Input: part model. Units: mm. Frame: model coordinates. Round coordinates to 2 decimals unless told otherwise and drop trailing zeros. Loops run counter-clockwise (first coordinate to the right, second up) from the corner with the lowest first, then second, coordinate; pieces in that order, holes last.
(1) Line query: line 1 (Y direction, x = -32, z = 10.75) (3 decimals); line 2 (Z direction, x = -163, y = -204); line 3 (Y direction, x = -152.5, z = 1) (3 decimals). Output: solid intervals per line, ascending.
(2) First-contact query: pin 1 Ø16 at (x, y) = (-15.92, -195.49) entering from -Z; pin 2 Ø3 at (x, y) = (-34, -167.5) entering from +Z; pin 3 Ø6.5 at (x, y) = (-86.2, -169.85) entering from +Z. Flat tips, straight axial feed; report the tip coordinate or a pass-through.
(3) Cut plane A-A, the plane x = -124.32. Output: boundary loops of the cut face in (y, z) (3 decimals), and give its area (3 significant figures).
from build123d import *

# Parameters (mm, degrees)
SKETCH1_W                                      = 184.15
SKETCH1_H                                      = 146.05
BOSS_EXTRUDE1_DEPTH                            = 12.7
SKETCH5_W                                      = 184.15
SKETCH5_H                                      = 12.7
BOSS_EXTRUDE2_DEPTH                            = 16.125
CBORE_FOR_M5_SHCS2_D                           = 5.8
CBORE_FOR_M5_SHCS2_CBORE_D                     = 10
CBORE_FOR_M5_SHCS2_CBORE_DEPTH                 = 5
CBORE_FOR_M5_SHCS3_D                           = 5.3
CBORE_FOR_M5_SHCS3_CBORE_D                     = 10
CBORE_FOR_M5_SHCS3_CBORE_DEPTH                 = 5
CBORE_START                                    = 5.3848
CBORE_SLOT_FOR_6_SOCKET_HEAD_CAP_SCREW1_DEPTH  = 7.3152
CBORE_SLOT_FOR_6_SOCKET_HEAD_CAP_SC_3_DEPTH    = 5.3848
CBORE_FOR_6_SOCKET_HEAD_CAP_SCREW1_D           = 4.3053
CBORE_FOR_6_SOCKET_HEAD_CAP_SCREW1_CBORE_D     = 7.14502
CBORE_FOR_6_SOCKET_HEAD_CAP_SCREW1_CBORE_DEPTH = 7.3152
F_8_CLEARANCE_HOLE1_D                          = 4.9149
CBORE_SLOT_FOR_6_SOCKET_HEAD_CAP_SCREW2_DEPTH  = 12.7
CBORE_START_2                                  = 7.9248
CBORE_SLOT_FOR_6_SOCKET_HEAD_CAP_SC_5_DEPTH    = 4.7752
SKETCH24_R                                     = 9.525
CUT_EXTRUDE2_DEPTH                             = 3.175
CUT_EXTRUDE3_REACH                             = 286.439
SKETCH25_R                                     = 3.96875
SKETCH26_R                                     = 9.525
CUT_EXTRUDE4_DEPTH                             = 5


# Read off the part's stored shape, not the designer's step: CBORE SLOT for #6 Socket Head Cap Screw1, CBORE SLOT for #6 Socket Head Cap Screw2
with BuildPart() as part:
    # Sketch1 → Boss-Extrude1 (new body)
    with BuildSketch(Plane.XY):
        with Locations((-90.01, -129)):
            Rectangle(SKETCH1_W, SKETCH1_H)
    extrude(amount=BOSS_EXTRUDE1_DEPTH)

    # Sketch5 → Boss-Extrude2 (add)
    with BuildSketch(Plane.XZ.offset(202.025)):
        with Locations((-90.01, 6.35)):
            Rectangle(SKETCH5_W, SKETCH5_H)
    extrude(amount=BOSS_EXTRUDE2_DEPTH)

    # CBORE for M5 SHCS2 (through all)
    with Locations(Plane.XY.offset(12.7)):
        with Locations((-55.7, -127.988675216), (-124.32, -127.988675216), (-90.01, -204.53125), (-143.810885302, -167.1), (-36.209114698, -167.1)):
            CounterBoreHole(CBORE_FOR_M5_SHCS2_D / 2, CBORE_FOR_M5_SHCS2_CBORE_D / 2, CBORE_FOR_M5_SHCS2_CBORE_DEPTH)

    # CBORE for M5 SHCS3 (through all)
    with Locations(Plane.XY.offset(12.7)):
        with Locations((-15.925, -65.5), (-15.925, -195.488675216), (-164.095, -195.488675216), (-163.361007118, -65.792154837)):
            CounterBoreHole(CBORE_FOR_M5_SHCS3_D / 2, CBORE_FOR_M5_SHCS3_CBORE_D / 2, CBORE_FOR_M5_SHCS3_CBORE_DEPTH)

    # CBORE SLOT for _6 Socket Head Cap Sc 2 → CBORE SLOT for #6 Socket Head Cap Screw1 (cut)
    with BuildSketch(Plane.XY.offset(CBORE_START)):
        with BuildLine():
            Line((-71.896135914, -174.858973451), (-71.896135914, -169.131273451))
            ThreePointArc((-71.896135914, -169.131273451), (-75.468645914, -165.558763451), (-79.041155914, -169.131273451))
            Line((-79.041155914, -169.131273451), (-79.041155914, -174.858973451))
            ThreePointArc((-79.041155914, -174.858973451), (-75.468645914, -178.431483451), (-71.896135914, -174.858973451))
        make_face()
        with BuildLine():
            Line((-100.978844086, -174.858973451), (-100.978844086, -169.131273451))
            ThreePointArc((-100.978844086, -169.131273451), (-104.551354086, -165.558763451), (-108.123864086, -169.131273451))
            Line((-108.123864086, -169.131273451), (-108.123864086, -174.858973451))
            ThreePointArc((-108.123864086, -174.858973451), (-104.551354086, -178.431483451), (-100.978844086, -174.858973451))
        make_face()
        with BuildLine():
            Line((-86.43749, -116.838826563), (-86.43749, -111.111126563))
            ThreePointArc((-86.43749, -111.111126563), (-90.01, -107.538616563), (-93.58251, -111.111126563))
            Line((-93.58251, -111.111126563), (-93.58251, -116.838826563))
            ThreePointArc((-93.58251, -116.838826563), (-90.01, -120.411336563), (-86.43749, -116.838826563))
        make_face()
    extrude(amount=CBORE_SLOT_FOR_6_SOCKET_HEAD_CAP_SCREW1_DEPTH, mode=Mode.SUBTRACT)

    # CBORE SLOT for _6 Socket Head Cap Sc 3 o → CBORE SLOT for _6 Socket Head Cap Sc 3 (cut)
    with BuildSketch(Plane.XY):
        with BuildLine():
            Line((-73.569995914, -174.858973451), (-73.569995914, -169.131273451))
            ThreePointArc((-73.569995914, -169.131273451), (-75.468645914, -167.232623451), (-77.367295914, -169.131273451))
            Line((-77.367295914, -169.131273451), (-77.367295914, -174.858973451))
            ThreePointArc((-77.367295914, -174.858973451), (-75.468645914, -176.757623451), (-73.569995914, -174.858973451))
        make_face()
        with BuildLine():
            Line((-102.652704086, -174.858973451), (-102.652704086, -169.131273451))
            ThreePointArc((-102.652704086, -169.131273451), (-104.551354086, -167.232623451), (-106.450004086, -169.131273451))
            Line((-106.450004086, -169.131273451), (-106.450004086, -174.858973451))
            ThreePointArc((-106.450004086, -174.858973451), (-104.551354086, -176.757623451), (-102.652704086, -174.858973451))
        make_face()
        with BuildLine():
            Line((-88.11135, -116.838826563), (-88.11135, -111.111126563))
            ThreePointArc((-88.11135, -111.111126563), (-90.01, -109.212476563), (-91.90865, -111.111126563))
            Line((-91.90865, -111.111126563), (-91.90865, -116.838826563))
            ThreePointArc((-91.90865, -116.838826563), (-90.01, -118.737476563), (-88.11135, -116.838826563))
        make_face()
    extrude(amount=CBORE_SLOT_FOR_6_SOCKET_HEAD_CAP_SC_3_DEPTH, mode=Mode.SUBTRACT)

    # CBORE for #6 Socket Head Cap Screw1 (through all)
    with Locations(Plane.XY.offset(12.7)):
        with Locations((-93.82, -169.850123451), (-86.2, -169.850123451)):
            CounterBoreHole(CBORE_FOR_6_SOCKET_HEAD_CAP_SCREW1_D / 2, CBORE_FOR_6_SOCKET_HEAD_CAP_SCREW1_CBORE_D / 2, CBORE_FOR_6_SOCKET_HEAD_CAP_SCREW1_CBORE_DEPTH)

    # #8 Clearance Hole1 (through all)
    with Locations(Plane.XY.offset(12.7)):
        with Locations((-32.01, -66.988675216), (-148.01, -66.988675216), (-148.01, -196.988675216), (-32.01, -196.988675216)):
            Hole(F_8_CLEARANCE_HOLE1_D / 2)

    # CBORE SLOT for _6 Socket Head Cap Sc 4 → CBORE SLOT for #6 Socket Head Cap Screw2 (cut)
    with BuildSketch(Plane.XY):
        with BuildLine():
            Line((-83.85735, -65.78485), (-83.85735, -60.56515))
            ThreePointArc((-83.85735, -60.56515), (-86.01, -58.4125), (-88.16265, -60.56515))
            Line((-88.16265, -60.56515), (-88.16265, -65.78485))
            ThreePointArc((-88.16265, -65.78485), (-86.01, -67.9375), (-83.85735, -65.78485))
        make_face()
        with BuildLine():
            Line((-91.85735, -85.78485), (-91.85735, -80.56515))
            ThreePointArc((-91.85735, -80.56515), (-94.01, -78.4125), (-96.16265, -80.56515))
            Line((-96.16265, -80.56515), (-96.16265, -85.78485))
            ThreePointArc((-96.16265, -85.78485), (-94.01, -87.9375), (-91.85735, -85.78485))
        make_face()
    extrude(amount=CBORE_SLOT_FOR_6_SOCKET_HEAD_CAP_SCREW2_DEPTH, mode=Mode.SUBTRACT)

    # CBORE SLOT for _6 Socket Head Cap Sc 5 o → CBORE SLOT for _6 Socket Head Cap Sc 5 (cut)
    # profile 1 of 2: a face of its own
    with BuildSketch(Plane.XY.offset(CBORE_START_2)):
        with BuildLine():
            Line((-82.43749, -65.78485), (-82.43749, -60.56515))
            ThreePointArc((-82.43749, -60.56515), (-86.01, -56.99264), (-89.58251, -60.56515))
            Line((-89.58251, -60.56515), (-89.58251, -65.78485))
            ThreePointArc((-89.58251, -65.78485), (-86.01, -69.35736), (-82.43749, -65.78485))
        make_face()
        with BuildLine():
            ThreePointArc((-88.16265, -60.56515), (-86.01, -58.4125), (-83.85735, -60.56515))
            Line((-83.85735, -60.56515), (-83.85735, -65.78485))
            ThreePointArc((-83.85735, -65.78485), (-86.01, -67.9375), (-88.16265, -65.78485))
            Line((-88.16265, -65.78485), (-88.16265, -60.56515))
        make_face(mode=Mode.SUBTRACT)
    # profile 2 of 2: a face of its own
    with BuildSketch(Plane.XY.offset(CBORE_START_2)):
        with BuildLine():
            Line((-90.43749, -85.78485), (-90.43749, -80.56515))
            ThreePointArc((-90.43749, -80.56515), (-94.01, -76.99264), (-97.58251, -80.56515))
            Line((-97.58251, -80.56515), (-97.58251, -85.78485))
            ThreePointArc((-97.58251, -85.78485), (-94.01, -89.35736), (-90.43749, -85.78485))
        make_face()
        with BuildLine():
            ThreePointArc((-96.16265, -80.56515), (-94.01, -78.4125), (-91.85735, -80.56515))
            Line((-91.85735, -80.56515), (-91.85735, -85.78485))
            ThreePointArc((-91.85735, -85.78485), (-94.01, -87.9375), (-96.16265, -85.78485))
            Line((-96.16265, -85.78485), (-96.16265, -80.56515))
        make_face(mode=Mode.SUBTRACT)
    extrude(amount=CBORE_SLOT_FOR_6_SOCKET_HEAD_CAP_SC_5_DEPTH, mode=Mode.SUBTRACT)

    # Sketch24 → Cut-Extrude2 (cut)
    with BuildSketch(Plane(origin=(0, 0, 0), x_dir=(-1, 0, 0), z_dir=(0, 0, -1))):
        with Locations((148.01, -66.988675216)):
            Circle(SKETCH24_R)
        with Locations((32.01, -66.988675216)):
            Circle(SKETCH24_R)
        with Locations((32.01, -196.988675216)):
            Circle(SKETCH24_R)
        with Locations((148.01, -196.988675216)):
            Circle(SKETCH24_R)
    extrude(amount=-CUT_EXTRUDE2_DEPTH, mode=Mode.SUBTRACT)

    # Sketch25 → Cut-Extrude3 (cut, up to next)
    with BuildSketch(Plane.XY.offset(12.7), mode=Mode.PRIVATE) as cut_extrude3_sk1:
        with Locations((-163.361007118, -65.792154837)):
            Circle(SKETCH25_R)
    cut_extrude3_tool1 = extrude(cut_extrude3_sk1.sketch, amount=-CUT_EXTRUDE3_REACH, mode=Mode.PRIVATE) & part.part
    # Sketch25 → Cut-Extrude3 (cut, up to next)
    with BuildSketch(Plane.XY.offset(12.7), mode=Mode.PRIVATE) as cut_extrude3_sk2:
        with Locations((-164.095, -195.488675216)):
            Circle(SKETCH25_R)
    cut_extrude3_tool2 = extrude(cut_extrude3_sk2.sketch, amount=-CUT_EXTRUDE3_REACH, mode=Mode.PRIVATE) & part.part
    add(cut_extrude3_tool1.solids().sort_by_distance((-163.361007, -65.792155, 12.7))[0], mode=Mode.SUBTRACT)
    add(cut_extrude3_tool2.solids().sort_by_distance((-164.095, -195.488675, 12.7))[0], mode=Mode.SUBTRACT)

    # Sketch26 → Cut-Extrude4 (cut)
    with BuildSketch(Plane.XY.offset(12.7)):
        with Locations((-164.095, -195.488675216)):
            Circle(SKETCH26_R)
        with Locations((-163.361007118, -65.792154837)):
            Circle(SKETCH26_R)
    extrude(amount=-CUT_EXTRUDE4_DEPTH, mode=Mode.SUBTRACT)


solid = part.part
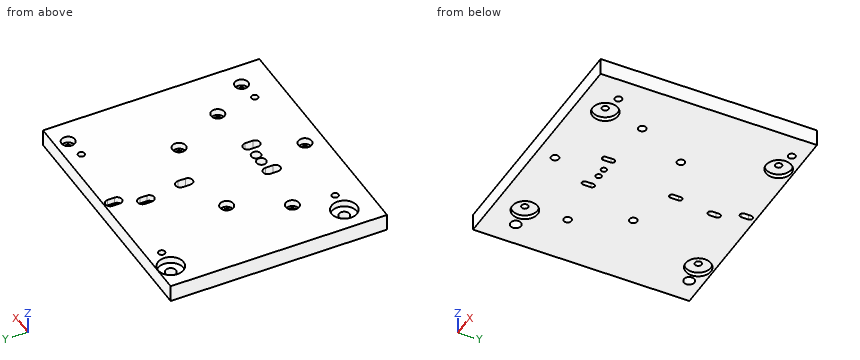
Reported:
1. line 1: y = -218.15 to -199.446, -194.531 to -169.799, -164.401 to -69.446, -64.531 to -55.975
1. line 2: z = 0 to 7.7
1. line 3: y = -218.15 to -205.389, -188.588 to -75.389, -58.588 to -55.975
2. pin 1: stops at z = 0
2. pin 2: stops at z = 7.7
2. pin 3: stops at z = 5.38
3. outline: (-218.15, 0) - (-130.889, 0) - (-130.889, 7.7) - (-132.989, 7.7) - (-132.989, 12.7) - (-218.15, 12.7) - close; (-125.089, 0) - (-55.975, 0) - (-55.975, 12.7) - (-122.989, 12.7) - (-122.989, 7.7) - (-125.089, 7.7) - close
3. area: 1,960 mm2
